For this review, take the finished solid that the model builds, in its own axes (mm). Give positions to 0.01 mm unless a question says otherwise; leave off trailing zeros. Write each loop counter-clockwise with the first axis right and the second up, starting at its lowest first coordinate (ties: lowest second). Pieces come first, ordered by that corner, then holes.
1) We need section B-B on y = -2. Give the boundary of the cut face in (x, z).
2) We need section A-A on x = 0. Give the boundary of the cut face in (y, z) (3 decimals), and give its area (3 significant figures).
3) We need section D-D on z = -0.3. Give the number of separate pieces and of enclosed holes in the cut face, and give its area (3 significant figures).
4) For P1, Ø3, axis at x = 14.38, y = 14.38, coming from the +Z side, flat-tipped, find the tip position at first contact; note if it passes through.
5) Wall thickness on line 1 along Y through (x, z) = (0, -0.15) (3 decimals); line 2 along X through (y, z) = (-11.5, -0.15); line 3 along X through (y, z) = (-15.5, -0.1): over which ranges is each line inside the solid? List them lowest first.
6) Draft analysis for pull direction X (two halves, no side actions). For faces 1 (the face through (-21.58, -11.11, -0.19)), 2 (the face through (12, 13, 0)), 3 (the face through (-3.555, 27.073, -0.188)), 4 (the face through (23.24, 12.64, -0.19)), state which applies: pulls with the +X half, pulls with the -X half, needs draft (parallel to the pull), parting line crosses it, or undercut.
7) We need section C-C on y = 15. Give the boundary of the cut face in (x, z), and give its area (3 significant figures).
from build123d import *

# Parameters (mm, degrees)
F0_R     = 27.305
F0_R_2   = 17.018
F1_DEPTH = 0.381
F2_D     = 2.9464
F3_D     = 3.5687


with BuildPart() as f1:
    # F0 (on Top) → F1 (new body)
    with BuildSketch(Plane.XY):
        Circle(F0_R)
        Circle(F0_R_2, mode=Mode.SUBTRACT)
    extrude(amount=-F1_DEPTH)

    # F2 (through all)
    with Locations(Plane.XY):
        with Locations((12.573, 21.7678), (21.7678, 12.573), (21.7678, -12.573), (12.573, -21.7678), (-12.573, -21.7678), (-21.7678, -12.573), (-21.7678, 12.573), (-12.573, 21.7678)):
            Hole(F2_D / 2)

    # F3 (through all)
    with Locations(Plane.XY):
        with Locations((14.3764, 14.3764), (14.3764, -14.3764), (-14.3764, -14.3764), (-14.3764, 14.3764)):
            Hole(F3_D / 2)


solid = f1.part
Results list:
1. outline: (-27.23, -0.38) - (-16.9, -0.38) - (-16.9, 0) - (-27.23, 0) - close; (16.9, -0.38) - (27.23, -0.38) - (27.23, 0) - (16.9, 0) - close
2. outline: (-27.305, -0.381) - (-17.018, -0.381) - (-17.018, 0) - (-27.305, 0) - close; (17.018, -0.381) - (27.305, -0.381) - (27.305, 0) - (17.018, 0) - close
2. area: 7.84 mm2
3. separate pieces: 1
3. enclosed holes: 13
3. area: 1,340 mm2
4. P1: passes through
5. line 1: y = -27.305 to -17.018, 17.018 to 27.305
5. line 2: x = -24.77 to -22.78, -20.76 to -12.54, 12.54 to 20.76, 22.78 to 24.77
5. line 3: x = -22.48 to -15.76, -12.99 to -7.03, 7.03 to 12.99, 15.76 to 22.48
6. face 1: undercut
6. face 2: needs draft
6. face 3: parting line crosses it
6. face 4: undercut
7. outline: (-22.82, -0.38) - (-16.05, -0.38) - (-16.05, 0) - (-22.82, 0) - close; (-12.7, -0.38) - (-8.04, -0.38) - (-8.04, 0) - (-12.7, 0) - close; (8.04, -0.38) - (12.7, -0.38) - (12.7, 0) - (8.04, 0) - close; (16.05, -0.38) - (22.82, -0.38) - (22.82, 0) - (16.05, 0) - close
7. area: 8.71 mm2
